CAD build for the part. Positions are in the model's coordinates, mm. Round coordinates to 2 decimals unless told otherwise and drop trailing zeros. Write each loop counter-clockwise with the first axis right and the second up, starting at its lowest first coordinate (ties: lowest second). Pieces come first, ordered by that corner, then holes. Notation, with made-up numbers: (69, -37) - (90, -37) arc R24 ccw to (90, -17) - close; hole circle Ø8 at (-25.5, 84). An arc over 180 degrees is marked (long way). Use one line per item in the form item = value. Start each with the question number.
Item 1: Band-saw the part on C-C, the plane x = 12. List the corners of the cut face in (y, z).
Item 2: Pin check, flat tip, straight feed: pin 1 (23.5 mm diameter, centred on x = 10.5, z = 7.5, fed in from +Y). Stop position of the tip, or through.
Item 3: Drill centre lines: L1, parallel to Z at x = -0.5, y = 0.15; L2, parallel to Y at x = 14.5, z = -13; L3, parallel to Z at x = -16, y = 0.15. Where is each one in solid material? Low to high.
from build123d import *

# Parameters (mm, degrees)
SKETCH1_R           = 20
BOSS_EXTRUDE1_DEPTH = 0.2
CUT_EXTRUDE1_DEPTH  = 29.284978345
CUT_EXTRUDE2_START  = -0.01
CUT_EXTRUDE2_DEPTH  = 0.01


with BuildPart() as part:
    # Sketch1 → Boss-Extrude1 (new body)
    with BuildSketch(Plane(origin=(0, 0, 0), x_dir=(1, 0, 0), z_dir=(0, 1, 0))):
        with Locations(Location((0, 0, 0), (0, 0, 270))):
            Circle(SKETCH1_R)
    extrude(amount=BOSS_EXTRUDE1_DEPTH)

    # Sketch2 → Cut-Extrude1 (cut, through all)
    with BuildSketch(Plane(origin=(0, 0.2, 0), x_dir=(1, 0, 0), z_dir=(0, 1, 0))):
        with BuildLine():
            Line((1.5, 19.5), (1.5, 19.943670675))
            ThreePointArc((1.5, 19.943670675), (0, 20), (-1.5, 19.943670675))
            Line((-1.5, 19.943670675), (-1.5, 19.5))
            Line((-1.5, 19.5), (-1, 19))
            Line((-1, 19), (1, 19))
            Line((1, 19), (1.5, 19.5))
        make_face()
    extrude(amount=-CUT_EXTRUDE1_DEPTH, mode=Mode.SUBTRACT)

    # Sketch3 → Cut-Extrude2 (cut)
    with BuildSketch(Plane(origin=(0, 0.2, 0), x_dir=(1, 0, 0), z_dir=(0, 1, 0)).offset(CUT_EXTRUDE2_START)):
        with BuildLine():
            ThreePointArc((-9.5, -17.599715907), (17.042589511, -10.466620408), (11.400670136, 16.432428927))
            Line((11.400670136, 16.432428927), (5.5, 9.400284093))
            Line((5.5, 9.400284093), (-9.5, 9.400284093))
            Line((-9.5, 9.400284093), (-9.5, -17.599715907))
        make_face()
    extrude(amount=CUT_EXTRUDE2_DEPTH, mode=Mode.SUBTRACT)


solid = part.part
Determined:
q1.outline = (0, -16) - (0.19, -16) - (0.19, 16) - (0, 16) - close
q2.pin_1 = 0.19
q3.L1 = -19 to 19.99
q3.L2 = 0 to 0.19
q3.L3 = -12 to 12
